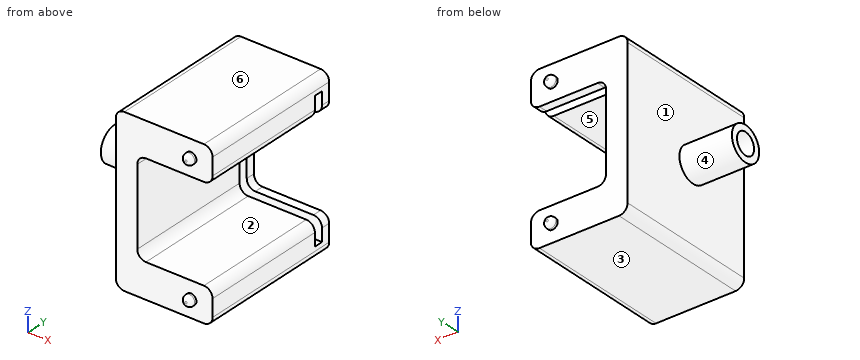
```python
from build123d import *

# Parameters (mm, degrees)
SALIENTE_EXTRUIR1_DEPTH = 30
REDONDEO1_R             = 2
CROQUIS2_R              = 4
SALIENTE_EXTRUIR2_DEPTH = 12.2
SALIENTE_EXTRUIR3_START = 2.1
SALIENTE_EXTRUIR3_DEPTH = 2.1
SALIENTE_EXTRUIR4_START = 2.1
SALIENTE_EXTRUIR4_DEPTH = 2.1
CROQUIS5_R              = 1.25
SALIENTE_EXTRUIR5_DEPTH = 1.5
REDONDEO2_R             = 1
SALIENTE_EXTRUIR6_START = 1.5
CROQUIS6_R              = 1.25
SALIENTE_EXTRUIR6_DEPTH = 1.5
REDONDEO3_R             = 1
CROQUIS7_R              = 2.5
CORTAR_EXTRUIR1_DEPTH   = 10


with BuildPart() as part:
    # Croquis1 → Saliente-Extruir1 (new body)
    with BuildSketch(Plane(origin=(0, 0, 0), x_dir=(1, 0, 0), z_dir=(0, 1, 0))):
        Polygon((0, 0), (22.5, 0), (22.5, 8), (5, 8), (5, 30), (22.5, 30), (22.5, 38), (0, 38), align=None)
    extrude(amount=SALIENTE_EXTRUIR1_DEPTH)

    # Redondeo1
    redondeo1_edges = [part.edges().sort_by_distance(p)[0] for p in [
        (0, 15, -38),
        (22.5, 15, -38),
        (22.5, 15, -30),
        (5, 15, -30),
        (5, 15, -8),
        (22.5, 15, -8),
        (22.5, 15, 0),
        (0, 15, 0),
    ]]
    fillet(redondeo1_edges, radius=REDONDEO1_R)

    # Croquis2 → Saliente-Extruir2 (add)
    with BuildSketch(Plane.ZY):
        with Locations(Location((-19, 15, 0), (0, 0, 180))):
            Circle(CROQUIS2_R)
    extrude(amount=SALIENTE_EXTRUIR2_DEPTH)

    # Croquis3 → Saliente-Extruir3 (add)
    with BuildSketch(Plane(origin=(0, 30, 0), x_dir=(1, 0, 0), z_dir=(0, 1, 0)).offset(SALIENTE_EXTRUIR3_START)):
        with BuildLine():
            Line((20.5, 38), (2, 38))
            ThreePointArc((2, 38), (0.585786438, 37.414213562), (0, 36))
            Line((0, 36), (0, 2))
            ThreePointArc((0, 2), (0.585786438, 0.585786438), (2, 0))
            Line((2, 0), (20.5, 0))
            ThreePointArc((20.5, 0), (21.914213562, 0.585786438), (22.5, 2))
            Line((22.5, 2), (22.5, 3))
            Line((22.5, 3), (3, 3))
            Line((3, 3), (3, 35))
            Line((3, 35), (22.5, 35))
            Line((22.5, 35), (22.5, 36))
            ThreePointArc((22.5, 36), (21.914213562, 37.414213562), (20.5, 38))
        make_face()
    extrude(amount=-SALIENTE_EXTRUIR3_DEPTH)

    # Croquis4 → Saliente-Extruir4 (add)
    with BuildSketch(Plane(origin=(0, 32.1, 0), x_dir=(1, 0, 0), z_dir=(0, 1, 0)).offset(SALIENTE_EXTRUIR4_START)):
        with BuildLine():
            Line((22.5, 32), (22.5, 36))
            ThreePointArc((22.5, 36), (21.914213562, 37.414213562), (20.5, 38))
            Line((20.5, 38), (2, 38))
            ThreePointArc((2, 38), (0.585786438, 37.414213562), (0, 36))
            Line((0, 36), (0, 2))
            ThreePointArc((0, 2), (0.585786438, 0.585786438), (2, 0))
            Line((2, 0), (20.5, 0))
            ThreePointArc((20.5, 0), (21.914213562, 0.585786438), (22.5, 2))
            Line((22.5, 2), (22.5, 6))
            ThreePointArc((22.5, 6), (21.914213562, 7.414213562), (20.5, 8))
            Line((20.5, 8), (7, 8))
            ThreePointArc((7, 8), (5.585786438, 8.585786438), (5, 10))
            Line((5, 10), (5, 28))
            ThreePointArc((5, 28), (5.585786438, 29.414213562), (7, 30))
            Line((7, 30), (20.5, 30))
            ThreePointArc((20.5, 30), (21.914213562, 30.585786438), (22.5, 32))
        make_face()
    extrude(amount=-SALIENTE_EXTRUIR4_DEPTH)

    # Croquis5 → Saliente-Extruir5 (add)
    with BuildSketch(Plane(origin=(0, 34.2, 0), x_dir=(1, 0, 0), z_dir=(0, 1, 0))):
        with Locations(Location((17.5, 34, 0), (0, 0, 270))):
            Circle(CROQUIS5_R)
        with Locations(Location((17.5, 4, 0), (0, 0, 90))):
            Circle(CROQUIS5_R)
    extrude(amount=SALIENTE_EXTRUIR5_DEPTH)

    # Redondeo2
    redondeo2_edges = [part.edges().sort_by_distance(p)[0] for p in [
        (17.5, 35.7, -35.25),
        (17.5, 35.7, -2.75),
    ]]
    fillet(redondeo2_edges, radius=REDONDEO2_R)

    # Croquis6 → Saliente-Extruir6 (add)
    with BuildSketch(Plane.XZ.offset(SALIENTE_EXTRUIR6_START)):
        with Locations(Location((17.5, -4, 0), (0, 0, 270))):
            Circle(CROQUIS6_R)
        with Locations(Location((17.5, -34, 0), (0, 0, 90))):
            Circle(CROQUIS6_R)
    extrude(amount=-SALIENTE_EXTRUIR6_DEPTH)

    # Redondeo3
    redondeo3_edges = [part.edges().sort_by_distance(p)[0] for p in [
        (17.5, -1.5, -2.75),
        (17.5, -1.5, -35.25),
    ]]
    fillet(redondeo3_edges, radius=REDONDEO3_R)

    # Croquis7 → Cortar-Extruir1 (cut)
    with BuildSketch(Plane.ZY.offset(12.2)):
        with Locations((-19, 15)):
            Circle(CROQUIS7_R)
    extrude(amount=-CORTAR_EXTRUIR1_DEPTH, mode=Mode.SUBTRACT)


solid = part.part
```
Source: CAD feature listing. Evaluate the final solid. Frame: model axes, mm. Face numbers are marked on the shaded views. A direction names the side the tool comes from. Give positions to 0.01 mm unless a question says otherwise; leave off trailing zeros. Write each loop counter-clockwise with the first axis right and the second up, starting at its lowest first coordinate (ties: lowest second). Pieces come first, ordered by that corner, then holes.
1. Section query C-C (z = -25.5). Return the cut outline in (x, y).
2. Material intervals for line 1 along Y through (x, z) = (-8, -19); line 2 along Y through (x, z) = (17.5, -7.5); line 3 along Z through (x, y) = (12.5, 28), sorted ascending.
3. Section query B-B (y = 5). Return the cut outline in (x, z).
4. Section query D-D (z = -19). Return the cut outline in (x, y), then the cut area to 3 significant figures.
5. First-contact query: pin 1 (2 mm diameter, centred on y = 6, z = -12.5, fed in from +X); pin 2 (3 mm diameter, centred on x = -5.5, y = 17.5, fed in from +Z); pin 3 (2 mm diameter, centred on x = -0.5, y = 28.5, fed in from -Z). Flat tips, straight axial feed; report the tip coordinate or a pass-through.
6. Section query A-A (x = 4). Return the cut outline in (y, z).
7. Pull-direction query (Z, two-part tool) for the marked faces 1, 2 and 3; classes: +Z half, -Z half, draft (parallel to the pull), parting line (faces both ways), or undercut.
8. Access query for the marked faces 4, 5 and 6. Directions: +Z, -Z, +X, -X, +Y, -Y. A direction counts if a zero-diameter tool reaches every point of the face in a straight line with its end or side. Return the directions, or none.
Output values:
1. outline: (0, 0) - (5, 0) - (5, 30) - (3, 30) - (3, 32.1) - (5, 32.1) - (5, 34.2) - (0, 34.2) - close
2. line 1: y = 11 to 12.5, 17.5 to 19
2. line 2: y = 0 to 30, 32.1 to 34.2
2. line 3: z = -38 to -30, -8 to 0
3. outline: (0, -36) arc R2 ccw to (2, -38) - (20.5, -38) arc R2 ccw to (22.5, -36) - (22.5, -32) arc R2 ccw to (20.5, -30) - (7, -30) arc R2 cw to (5, -28) - (5, -10) arc R2 cw to (7, -8) - (20.5, -8) arc R2 ccw to (22.5, -6) - (22.5, -2) arc R2 ccw to (20.5, 0) - (2, 0) arc R2 ccw to (0, -2) - close
4. outline: (-12.2, 11) - (0, 11) - (0, 0) - (5, 0) - (5, 30) - (3, 30) - (3, 32.1) - (5, 32.1) - (5, 34.2) - (0, 34.2) - (0, 19) - (-12.2, 19) - (-12.2, 17.5) - (-2.2, 17.5) - (-2.2, 12.5) - (-12.2, 12.5) - close
4. area: 214 mm2
5. pin 1: stops at x = 5
5. pin 2: stops at z = -15.13
5. pin 3: stops at z = -37.32
6. outline: (0, -38) - (34.2, -38) - (34.2, 0) - (0, 0) - close; hole (30, -35) - (32.1, -35) - (32.1, -3) - (30, -3) - close
7. face 1: draft
7. face 2: undercut
7. face 3: -Z half
8. face 4: -X
8. face 5: +X, +Y, -Y
8. face 6: +Z, +X, -X, +Y, -Y
